```python
from build123d import *

# Parameters (mm, degrees)
BOSS_EXTRUDE1_DEPTH = 2
SKETCH2_R           = 10
BOSS_EXTRUDE2_DEPTH = 6
CUT_EXTRUDE1_DEPTH  = 2


with BuildPart() as part:
    # Sketch1 → Boss-Extrude1 (new body)
    with BuildSketch(Plane.XY):
        Polygon((-2.571996213, -4.179493846), (2.333549739, -4.317160982), (4.905545953, -0.137667136), (2.571996213, 4.179493846), (-2.333549739, 4.317160982), (-4.905545953, 0.137667136), align=None)
        Polygon((2.208890865, 3.589447656), (-2.004107423, 3.707679432), (-4.212998289, 0.118231775), (-2.208890865, -3.589447656), (2.004107423, -3.707679432), (4.212998289, -0.118231775), align=None, mode=Mode.SUBTRACT)
    extrude(amount=BOSS_EXTRUDE1_DEPTH)

    # Sketch2 → Boss-Extrude2 (add)
    with BuildSketch(Plane.XY.offset(2)):
        Circle(SKETCH2_R)
    extrude(amount=BOSS_EXTRUDE2_DEPTH)

    # Sketch5 → Cut-Extrude1 (cut)
    with BuildSketch(Plane(origin=(0, 0, 2), x_dir=(-1, 0, 0), z_dir=(0, 0, -1))):
        Polygon((-2.208890865, 3.589447656), (-4.212998289, -0.118231775), (-2.004107423, -3.707679432), (2.208890865, -3.589447656), (4.212998289, 0.118231775), (2.004107423, 3.707679432), align=None)
    extrude(amount=-CUT_EXTRUDE1_DEPTH, mode=Mode.SUBTRACT)


solid = part.part
```
The listing builds one solid part. Answer for the finished solid, in the listing's coordinates (mm). A direction names the side the tool comes from. Round coordinates to 2 decimals unless told otherwise and drop trailing zeros. Loops run counter-clockwise (first coordinate to the right, second up) from the corner with the lowest first, then second, coordinate; pieces in that order, holes last. Notation, with made-up numbers: (86.5, 63) -> (114.5, 63) arc R33 ccw to (114.5, 102) -> close; hole circle Ø8 at (-27.75, 71.5). An arc over 180 degrees is marked (long way). Use one line per item in the form item = value.
1. Flat-ended cylindrical pins translate along their axes: pin 1 Ø1.5 at (y, z) = (4.5, 1.5) entering from +X; pin 2 Ø3 at (y, z) = (-4.5, 1.5) entering from +X; pin 3 Ø1 at (y, z) = (6.5, 5) entering from +X. Find the tip coordinate at first contact, or state that the pin passes through.
Answer key:
pin_1 = 9.19
pin_2 = 9.51
pin_3 = 8
2. The part is cut by section B-B on y = -1.5. Determine the outline of the cut face in (x, z), and give its area (3 significant figures).
Answer key:
outline = (-9.89, 2) -> (-4.02, 2) -> (-4.02, 0) -> (-3.34, 0) -> (-3.34, 4) -> (3.36, 4) -> (3.36, 0) -> (4.07, 0) -> (4.07, 2) -> (9.89, 2) -> (9.89, 8) -> (-9.89, 8) -> close
area = 108 mm²
3. A tool of negligible diameter and unlimited length cuts with its end or side. For faces 1 (the flat face through (-3.755, -1.991, 0.986)), 2 (the flat face through (-3.6, 2.26, 0.99)), 3 (the flat face through (3.225, 1.71, 1.972)), 4 (the flat face through (3.6, -2.26, 0.99)), from which of +Z, -Z, +X, -X, +Y, -Y can it reach the whole face along a straight path? Write none if from no direction.
Answer key:
face_1 = -Z, -X, -Y
face_2 = -Z, -X, +Y
face_3 = -Z
face_4 = -Z, +X, -Y
4. The part is cut by section C-C on x = -3.25. Determine the outline of the cut face in (y, z), and give its area (3 significant figures).
Answer key:
outline = (-9.46, 2) -> (-2.93, 2) -> (-2.93, 0) -> (-1.66, 0) -> (-1.66, 4) -> (1.68, 4) -> (1.68, 0) -> (2.83, 0) -> (2.83, 2) -> (9.46, 2) -> (9.46, 8) -> (-9.46, 8) -> close
area = 112 mm²
5. The part is cut by section A-A on z = 2.5. Determine the outline of the cut face in (x, y).
Answer key:
outline = circle Ø20 at (0, 0); hole (-4.21, 0.12) -> (-2.21, -3.59) -> (2, -3.71) -> (4.21, -0.12) -> (2.21, 3.59) -> (-2, 3.71) -> close
6. Find the intervals of material crossed by probe 1 along Z at (x, y) = (1.75, 5); probe 2 along Y at (x, z) = (-2.5, 1.25); probe 3 along Z at (x, y) = (-0.25, 3.5), in increasing order. Write a range as [from, to].
Answer key:
probe_1 = [2, 8]
probe_2 = [-4.18, -3.05], [2.9, 4.05]
probe_3 = [4, 8]
7. The part is cut by section D-D on z = 5. Determine the outline of the cut face in (x, y).
Answer key:
outline = circle Ø20 at (0, 0)
8. For a pull along X with two mould halves and no side action, classify faces 5 (the cylindrical face through (-2.17, -9.76, 4.96)), 6 (the flat face through (0, 0, 8)), 7 (the flat face through (-3.225, -1.71, 1.972)) as released by +X, released by -X, zero draft, split by the parting line, or undercut.
Answer key:
face_5 = split by the parting line
face_6 = zero draft
face_7 = undercut
